Part model, mm, in its own coordinate system. A direction names the side the tool comes from. Give positions to 0.01 mm unless a question says otherwise; leave off trailing zeros. Write each loop counter-clockwise with the first axis right and the second up, starting at its lowest first coordinate (ties: lowest second). Pieces come first, ordered by that corner, then holes. Notation, with made-up numbers: M -20,49 L -10,49 A30 ccw -10,73 Z; hole C 30.5,79 d3. An arc over 180 degrees is marked long. Use CSV: the item, a comma, the result in double quotes. Start each with the question number.
1. Band-saw the part on B-B, the plane z = 0. List the corners of the cut face in (x, y).
2. Band-saw the part on C-C, the plane z = 10.16. List the corners of the cut face in (x, y) (3 decimals), then the cut area to 3 significant figures.
3. Drill centre lines: line 1 along X through (y, z) = (4.5, 0); line 2 along Y through (x, z) = (5.25, 4.75); line 3 along Y through (x, z) = (-0.5, 8). Where is each one in solid material? Low to high. Write a range as from..to.
4. Band-saw the part on D-D, the plane y = 3. List the corners of the cut face in (x, z), then the cut area to 3 significant figures.
5. 3-axis set-ups, long thin cutter, end or side, ignore diameter. For faces 4 (the face through (0, 8, -5.644)), 5 (the face through (0, 0, 0)), 6 (the face through (6.943, 1.656, 1.542)): which of +Z, -Z, +X, -X, +Y, -Y reach the whole face in a straight line?
6. Drop flat-ended pins along their axis: pin 1 Ø3.5 at (x, z) = (0, -9.5) entering from +Y (3 decimals); pin 2 Ø1 at (x, z) = (0, 10.5) entering from +Y; pin 3 Ø0.5 at (x, y) = (0, 7) entering from -Z. Give the stop position or say it passes through.
7. Band-saw the part on A-A, the plane y = 6. List the corners of the cut face in (x, z).
8. Mould opens along X. For faces 1 (the face through (0, 7, 6)), 2 (the face through (0, 1.27, -10)), 3 (the face through (-5, 2.032, 4)) say: pulls with the +X half, pulls with the -X half, needs draft (parallel to the pull), parting line crosses it, or undercut.
Autodesk Inventor part; units mm, degrees
ref_plane "hex_face_nut_XY" through (0, 2.032, 0) normal (0, 1, 0) x (1, 0, 0)
ref_plane "hex_face_nut_YZ" through (0, 2.032, 0) normal (1, 0, 0) x (0, 0, -1)
ref_plane "hex_face_nut_ZX" through (0, 2.032, 0) normal (0, 0, -1) x (0, 1, 0)
sketch "Sketch_1" plane through (0, 0, 0) normal (0, 1, 0) x (-1, 0, 0)
  line L0 (7.874, -12.7) -> (7.874, 12.7)
  arc A0 (7.874, 12.7) -> (7.366, 13.208) centre (7.366, 12.7) ccw
  line L1 (7.366, 13.208) -> (-7.366, 13.208)
  arc A1 (-7.366, 13.208) -> (-7.874, 12.7) centre (-7.366, 12.7) ccw
  line L2 (-7.874, 12.7) -> (-7.874, -12.7)
  arc A2 (-7.874, -12.7) -> (-7.366, -13.208) centre (-7.366, -12.7) ccw
  line L3 (-7.366, -13.208) -> (7.366, -13.208)
  arc A3 (7.366, -13.208) -> (7.874, -12.7) centre (7.366, -12.7) ccw
extrude "Extrusion1" add sketch "Sketch_1" along normal blind 1.27
sketch "Sketch_4" plane through (0, 0, 0) normal (1, 0, 0) x (0, 1, 0)
  line L0 (0.762, 0) -> (11.9126, 0)
  line L1 (11.9126, -3.7592) -> (0.762, -3.7592)
  line L2 (0.762, -3.7592) -> (0.762, -7.112)
  line L3 (0.762, -7.112) -> (2.032, -7.112)
  line L4 (2.032, -7.112) -> (2.032, -6)
  line L5 (2.032, -6) -> (11.2991, -6)
  line L6 (11.2991, -6) -> (11.9126, -5.3865)
  line L7 (11.9126, -5.3865) -> (11.9126, -3.7592)
revolve "Revolution1" add sketch "Sketch_4" angle 360 about axis through (0, 0.762, 0) along (0, -1, 0)
thread "Thread1"
sketch "Sketch_6" plane through (0, 3.81, 0) normal (0, 1, 0) x (1, 0, 0)
  line L0 (-0.508, 5.6444) -> (0.508, 5.6444)
  line L1 (0.508, 5.6444) -> (0.508, 6.4064)
  line L2 (0.508, 6.4064) -> (-0.508, 6.4064)
  line L3 (-0.508, 6.4064) -> (-0.508, 5.6444)
extrude "Extrusion2" cut sketch "Sketch_6" along normal blind 25.4
sketch "Sketch_2" plane through (0, 0, -10.16) normal (0, 0, 1) x (1, 0, 0)
  line L0 (0, 1.27) -> (0, 1.905)
  line L1 (1.25, 1.27) -> (2, 1.27)
  line L2 (2, 1.27) -> (2, 1.524)
  arc A0 (2, 1.524) -> (1.619, 1.905) centre (1.619, 1.524) ccw
  line L3 (1.619, 1.905) -> (1.25, 1.905)
  line L4 (1.25, 1.905) -> (1.25, 1.27)
revolve "Revolution2" add sketch "Sketch_2" angle 360 about axis through (0, 1.27, -10.16) along (0, -1, 0)
sketch "Sketch_3" plane through (0, 0, 10.16) normal (0, 0, 1) x (1, 0, 0)
  line L0 (0, 1.27) -> (0, 1.905)
  line L1 (1.25, 1.27) -> (2, 1.27)
  line L2 (2, 1.27) -> (2, 1.524)
  arc A0 (2, 1.524) -> (1.619, 1.905) centre (1.619, 1.524) ccw
  line L3 (1.619, 1.905) -> (1.25, 1.905)
  line L4 (1.25, 1.905) -> (1.25, 1.27)
revolve "Revolution3" add sketch "Sketch_3" angle 360 about axis through (0, 1.27, 10.16) along (0, -1, 0)
ref_plane "hex_face_nut_XY" through (0, 2.032, 0) normal (0, 1, 0) x (1, 0, 0)
ref_plane "hex_face_nut_YZ" through (0, 2.032, 0) normal (1, 0, 0) x (0, 0, -1)
ref_plane "hex_face_nut_ZX" through (0, 2.032, 0) normal (0, 0, -1) x (0, 1, 0)
ref_plane "knurled_nut_XY" through (0, 4.5466, 0) normal (0, 1, 0) x (1, 0, 0)
ref_plane "knurled_nut_YZ" through (0, 4.5466, 0) normal (1, 0, 0) x (0, 0, -1)
ref_plane "knurled_nut_ZX" through (0, 4.5466, 0) normal (0, 0, -1) x (0, 1, 0)
ref_plane "lockwasher_XY" through (0, 4.0386, 0) normal (0, 1, 0) x (1, 0, 0)
ref_plane "lockwasher_YZ" through (0, 4.0386, 0) normal (1, 0, 0) x (0, 0, -1)
ref_plane "lockwasher_ZX" through (0, 4.0386, 0) normal (0, 0, -1) x (0, 1, 0)
ref_plane "panel_XY" through (0, 0, 0) normal (0, -1, 0) x (1, 0, 0)
ref_plane "panel_YZ" through (0, 0, 0) normal (1, 0, 0) x (0, 0, 1)
ref_plane "panel_ZX" through (0, 0, 0) normal (0, 0, 1) x (0, -1, 0)
ref_plane "toggle_XY" through (0, 9.4107, 0) normal (0, 1, 0) x (1, 0, 0)
ref_plane "toggle_YZ" through (0, 9.4107, 0) normal (1, 0, 0) x (0, 0, -1)
ref_plane "toggle_ZX" through (0, 9.4107, 0) normal (0, 0, -1) x (0, 1, 0)
properties part number "SS114-panel"
Output:
1,outline,"M -7.87,0 L 7.87,0 L 7.87,1.27 L 7.11,1.27 L 7.11,2.03 L 6,2.03 L 6,11.3 L 5.39,11.91 L 3.76,11.91 L 3.76,1.27 L -3.76,1.27 L -3.76,11.91 L -5.39,11.91 L -6,11.3 L -6,2.03 L -7.11,2.03 L -7.11,1.27 L -7.87,1.27 Z"
2,outline,"M -7.874,0 L 7.874,0 L 7.874,1.27 L 2,1.27 L 2,1.524 A0.381 ccw 1.619,1.905 L 1.25,1.905 L 1.25,1.27 L -1.25,1.27 L -1.25,1.905 L -1.619,1.905 A0.381 ccw -2,1.524 L -2,1.27 L -7.874,1.27 Z"
2,area,"20.9 mm²"
3,line 1,"x = -6..-3.76, 3.76..6"
3,line 2,"y = 0..2.03"
3,line 3,"y = 0..1.27"
4,outline,"C 0,0 d12; hole C 0,0 d7.52"
4,area,"68.7 mm²"
5,face 4,"-Z, +Y"
5,face 5,"+Z, -Z, +X, -X, -Y"
5,face 6,"+Y"
6,pin 1,"stops at y = 1.905"
6,pin 2,"stops at y = 1.27"
6,pin 3,"stops at z = -5.64"
7,outline,"M -0.51,-5.98 L -0.51,-5.64 L 0.51,-5.64 L 0.51,-5.98 A6 ccw long Z; hole C 0,0 d7.52"
8,face 1,"parting line crosses it"
8,face 2,"undercut"
8,face 3,"needs draft"
